Autodesk Inventor part; units mm, degrees
ref_plane "YZ Plane" through (0, 0, 0) normal (1, 0, 0) x (0, 1, 0)
ref_plane "XZ Plane" through (0, 0, 0) normal (0, 1, 0) x (-1, 0, 0)
ref_plane "XY Plane" through (0, 0, 0) normal (0, 0, 1) x (1, 0, 0)
sketch "Szkic1" plane through (0, 0, 0) normal (0, 0, 1) x (1, 0, 0)
  line L0 (0, 0) -> (25, 0)
  line L1 (25, 0) -> (25, 5)
  line L2 (25, 5) -> (0, 5)
  line L3 (0, 5) -> (0, 0)
  line L4 (0, 5) -> (25, 5)
  line L5 (25, 5) -> (25, 25)
  line L6 (25, 25) -> (0, 25)
  line L7 (0, 25) -> (0, 5)
  dimension "d0" = 5
  dimension "d1" = 25
  dimension "d2" = 20
extrude "Wyciągnięcie proste1" add sketch "Szkic1" along normal blind 5 contours L7 L6 L5 L2
extrude "Wyciągnięcie proste2" add sketch "Szkic1" along normal blind 25 contours L3 L2 L1 L0
chamfer "Faza1" distance 5 angle 45 1 edges at (12.5, 5, 5)
sketch "Szkic2" plane through (0, 5, 25) normal (0, 1, 0) x (1, 0, 0)
  line L0 (0, 15) -> (25, 15)
  line L1 (0, 15) -> (0, 0)
  line L2 (25, 0) -> (0, 0)
  line L3 (25, 15) -> (25, 0)
  line L4 (25, 0) -> (0, 0)
  line L5 (12.5, 0) -> (12.5, 15)
  circle A0 centre (7.5, 7.5) radius 2.6
  circle A1 centre (17.5, 7.5) radius 2.6
  point P0 (0, 25)
  dimension "d10" = 5.2
  dimension "d11" = 10
  dimension "d12" = 7.5
  dimension "d21" = 15
extrude "Wyciągnięcie proste3" cut sketch "Szkic2" against normal up to surface (5 mm away) contours A0 | A1
sketch "Szkic3" plane through (0, 0, 5) normal (0, 0, 1) x (1, 0, 0)
  line L0 (25, 10) -> (0, 10)
  line L1 (25, 10) -> (25, 25)
  line L2 (25, 25) -> (0, 25)
  line L3 (0, 25) -> (0, 10)
  circle A0 centre (17.5, 17.5) radius 2.6
  circle A1 centre (7.5, 17.5) radius 2.6
  line L4 (25, 25) -> (0, 25)
  line L5 (12.5, 25) -> (12.5, 10)
  point P0 (0, 0)
  dimension "d15" = 5.2
  dimension "d16" = 10
  dimension "d20" = 7.5
  dimension "d22" = 15
extrude "Wyciągnięcie proste4" cut sketch "Szkic3" against normal up to surface (5 mm away) contours A0 | A1
fillet "Zaokrąglenie1" radius 1.6 7 edges at (12.5, 0, 0) (12.5, 0, 25) (12.5, 5, 25) (12.5, 5, 10) (12.5, 10, 5) (12.5, 25, 5) (12.5, 25, 0)
equation "\"d12\" = 0.5 * d21"
equation "\"d20\" = 0.5 * d22"
properties part number "motor_rig_v2"
For this review, take the finished solid that the model builds, in its own axes (mm). A direction names the side the tool comes from. Round coordinates to 2 decimals unless told otherwise and drop trailing zeros. Loops run counter-clockwise (first coordinate to the right, second up) from the corner with the lowest first, then second, coordinate; pieces in that order, holes last. Notation, with made-up numbers: (25.5, -39.5) - (29.5, -39.5) arc R15 cw to (29.5, -11.5) - close; hole circle Ø2 at (25, -33). An arc over 180 degrees is marked (long way). Put each result on its own line as item: value. Start each with the question number.
1. For probe 1 along X at (y, z) = (2.6, 17.5); probe 2 along Y at (x, z) = (17.5, 2.45), list the stretches that pass through material, from the lowest coordinate up. Write a range as [from, to].
2. For faces 1 (the flat face through (13, 5, 17)), 2 (the cylindrical face through (12.68, 0.48, 24.54)), list the 3-axis set-ups (+Z, -Z, +X, -X, +Y, -Y) from which the entire face can be reached by the end or side of a thin tool; tool diameter is ignored.
3. Insertion check: P1, Ø8, axis at x = 22.5, y = 17.5, coming from the +Z side; P2, Ø2, axis at x = 20, z = 13.5, coming from the -Y side; P3, Ø14, axis at x = 14, z = 20, coming from the +Y side. Each pin has a flat end and moves straight along its axis. Give the tip position at first contact, or say it passes through.
4. Consider section D-D on x = 3. State the section outline as (y, z) points.
5. Consider section A-A on x = 17.5. State the section outline as (y, z) points, plus the area to 3 significant figures.
6. Consider section B-B on y = 17.5. State the section outline as (x, z) points.
7. Mouldability with a two-part tool opening along Z and no side actions: class faces 3 (the flat face through (0, 7, 7)), 4 (the cylindrical face through (9.9, 2.5, 18.5)), 5 (the cylindrical face through (19.9, 2.5, 18.5)), 6 (the flat face through (12, 13, 0)) as +Z half, -Z half, draft (parallel to the pull), parting line (faces both ways), or undercut.
Result sheet:
1. probe 1: [0, 4.9], [10.1, 14.9], [20.1, 25]
1. probe 2: [0, 14.9], [20.1, 25]
2. face 1: +Z, +X, -X, +Y
2. face 2: +Z, +X, -X, -Y
3. P1: z = 5
3. P2: y = 0
3. P3: y = 5
4. outline: (0, 1.6) arc R1.6 ccw to (1.6, 0) - (23.4, 0) arc R1.6 ccw to (25, 1.6) - (25, 3.4) arc R1.6 ccw to (23.4, 5) - (10.66, 5) arc R1.6 cw to (9.53, 5.47) - (5.47, 9.53) arc R1.6 cw to (5, 10.66) - (5, 23.4) arc R1.6 ccw to (3.4, 25) - (1.6, 25) arc R1.6 ccw to (0, 23.4) - close
5. outline: (0, 1.6) arc R1.6 ccw to (1.6, 0) - (14.9, 0) - (14.9, 5) - (10.66, 5) arc R1.6 cw to (9.53, 5.47) - (5.47, 9.53) arc R1.6 cw to (5, 10.66) - (5, 14.9) - (0, 14.9) - close; (0, 20.1) - (5, 20.1) - (5, 23.4) arc R1.6 ccw to (3.4, 25) - (1.6, 25) arc R1.6 ccw to (0, 23.4) - close; (20.1, 0) - (23.4, 0) arc R1.6 ccw to (25, 1.6) - (25, 3.4) arc R1.6 ccw to (23.4, 5) - (20.1, 5) - close
5. area: 183 mm^2
6. outline: (0, 0) - (4.9, 0) - (4.9, 5) - (0, 5) - close; (10.1, 0) - (14.9, 0) - (14.9, 5) - (10.1, 5) - close; (20.1, 0) - (25, 0) - (25, 5) - (20.1, 5) - close
7. face 3: draft
7. face 4: undercut
7. face 5: undercut
7. face 6: -Z half
